The listing builds one solid part. Answer for the finished solid, in the listing's coordinates (mm). A direction names the side the tool comes from. Round coordinates to 2 decimals unless told otherwise and drop trailing zeros. Write each loop counter-clockwise with the first axis right and the second up, starting at its lowest first coordinate (ties: lowest second). Pieces come first, ordered by that corner, then holes. Notation, with made-up numbers: (76.5, 82) - (96.5, 82) arc R16 cw to (96.5, 109) - close; hole circle Ø7 at (-30.5, -10.5). An arc over 180 degrees is marked (long way). Use a Markdown table: item, result. Add a question column.
1) A tool of negligible diameter and unlimited length cuts with its end or side. For faces 1 (the cylindrical face through (20.544, 17.244, 72.039)), 2 (the flat face through (17.7, 22, 79.798)), from which of +Z, -Z, +X, -X, +Y, -Y can it reach the whole face along a straight path? Write none if from no direction.
2) A cutting plane is placed at A-A (y = 15.25). Give the vertices of the cut face in (x, z), then the cut area to 3 significant figures.
3) A cutting plane is placed at D-D (z = 20). Give the vertices of the cut face in (x, y) (1 decimal), then the cut area to 3 significant figures.
4) Determine the mould class of faces 3 (the flat face through (20, 20, 0)), 4 (the cylindrical face through (12.242, 13.735, 39.341)), 5 (the conical face through (20.24, 20.05, 70.06)) for opening direction Y: +Y half, -Y half, draft (parallel to the pull), parting line (faces both ways), or undercut.
5) Find the intervals of material crossed by probe 1 along Y at (x, z) = (20.5, 76); probe 2 along Y at (x, z) = (19.25, 75.5) (3 decimals); probe 3 along X at (y, z) = (16, 14.5), in increasing order. Write a range as from..to.
6) A cutting plane is placed at C-C (z = 74). Give the vertices of the cut face in (x, y) (1 decimal), then the cut area to 3 significant figures.
7) Each of these flat-tipped pins is pushed along its axis until it touches: P1, Ø8, axis at x = 12.5, z = 41, coming from the +Y side; P2, Ø1, axis at y = 27, z = 21.5, coming from the +X side; P3, Ø4, axis at x = 20, y = 19.68, coming from the +Z side. Where does it stop, or does it pass through?
8) A cutting plane is placed at B-B (x = 23.75). Give the vertices of the cut face in (y, z).
```python
from build123d import *

# Parameters (mm, degrees)
SKETCH1_R                   = 9.779
BOSS_EXTRUDE1_DEPTH         = 92.6
SKETCH2_R                   = 3.4925
CUT_EXTRUDE1_DEPTH          = 30.7815
FILLET1_R                   = 0.254
FILLET2_R                   = 0.254
SKETCH3_R                   = 11.060223395
CUT_EXTRUDE2_DEPTH          = 12.8016
M6_TAPPED_HOLE1_D           = 5
M6_TAPPED_HOLE1_DEPTH       = 8.497848452
M6_TAPPED_HOLE1_CBORE_D     = 6
M6_TAPPED_HOLE1_CBORE_DEPTH = 7
M6_TAPPED_HOLE1_TIP         = 1.502151548


with BuildPart() as part:
    # Sketch1 → Boss-Extrude1 (new body)
    with BuildSketch(Plane.XY):
        with Locations((20.0025, 19.685)):
            Circle(SKETCH1_R)
    extrude(amount=BOSS_EXTRUDE1_DEPTH)

    # Sketch2 → Cut-Extrude1 (cut, through all)
    with BuildSketch(Plane(origin=(0, 0, 0), x_dir=(0, 0, -1), z_dir=(1, 0, 0))):
        with Locations((-83.583, 19.685)):
            Circle(SKETCH2_R)
    extrude(amount=CUT_EXTRUDE1_DEPTH, mode=Mode.SUBTRACT)

    # Fillet1
    fillet1_edges = [part.edges().sort_by_distance(p)[0] for p in [
        (29.136572736, 23.1775, 83.583),
        (10.2235, 19.685, 87.075500001),
    ]]
    fillet(fillet1_edges, radius=FILLET1_R)

    # Fillet2
    fillet2_edges = [part.edges().sort_by_distance(p)[0] for p in [
        (10.2235, 19.685, 92.6),
    ]]
    fillet(fillet2_edges, radius=FILLET2_R)

    # Sketch3 → Cut-Extrude2 (cut)
    with BuildSketch(Plane.XY.offset(92.6)):
        with Locations((20.0025, 19.685)):
            Circle(SKETCH3_R)
    extrude(amount=-CUT_EXTRUDE2_DEPTH, mode=Mode.SUBTRACT)

    # M6 Tapped Hole1
    with Locations(Plane(origin=(20.0025, 19.685, 79.7984), x_dir=(1, 0, 0), z_dir=(0, 0, 1))):
        with Locations((0, 0)):
            CounterBoreHole(M6_TAPPED_HOLE1_D / 2, M6_TAPPED_HOLE1_CBORE_D / 2, M6_TAPPED_HOLE1_CBORE_DEPTH, depth=M6_TAPPED_HOLE1_DEPTH)
            with Locations((0, 0, -(M6_TAPPED_HOLE1_DEPTH + M6_TAPPED_HOLE1_TIP / 2))):  # 118° drill point
                Cone(0, M6_TAPPED_HOLE1_D / 2, M6_TAPPED_HOLE1_TIP, mode=Mode.SUBTRACT)


solid = part.part
```
Entries:
| question | item | result |
|---|---|---|
| 1 | face 1 | +Z |
| 1 | face 2 | +Z, +X, -X, +Y, -Y |
| 2 | outline | (11.29, 0) - (28.72, 0) - (28.72, 79.8) - (11.29, 79.8) - close |
| 2 | area | 1,390 mm² |
| 3 | outline | circle Ø19.6 at (20, 19.7) |
| 3 | area | 300 mm² |
| 4 | face 3 | draft |
| 4 | face 4 | parting line |
| 4 | face 5 | undercut |
| 5 | probe 1 | y = 9.92..16.73, 22.64..29.45 |
| 5 | probe 2 | y = 9.935..16.781, 22.589..29.435 |
| 5 | probe 3 | x = 10.94..29.06 |
| 6 | outline | circle Ø19.6 at (20, 19.7); hole circle Ø6 at (20, 19.7) |
| 6 | area | 272 mm² |
| 7 | P1 | stops at y = 28.82 |
| 7 | P2 | stops at x = 27.02 |
| 7 | P3 | stops at z = 71 |
| 8 | outline | (10.65, 0) - (28.72, 0) - (28.72, 79.8) - (10.65, 79.8) - close |
